The drawing under review shows one solid part. Ordinate dimensions are in mm from its lowest x, y, z. A direction names the side the tool comes from. Give positions to 0.01 mm unless a question says otherwise; leave off trailing zeros. Loops run counter-clockwise (first coordinate to the right, second up) from the corner with the lowest first, then second, coordinate; pieces in that order, holes last. Notation, with made-up numbers: M 37.5,19.5 L 92.5,19.5 A23 cw 92.5,45.5 Z; hole C 0,28 d9. An arc over 180 degrees is marked long. Write item = value, one per line. Start each with the question number.
1. For the marked faces 4, 5 and 6, list the 3-axis set-ups (+Z, -Z, +X, -X, +Y, -Y) from which the entire face can be reached by the end or side of a thin tool; tool diameter is ignored.
2. Draft analysis for pull direction Z (two halves, no side actions). For the marked faces 1, 2 and 3, state which applies: pulls with the +Z half, pulls with the -Z half, needs draft (parallel to the pull), parting line crosses it, or undercut.
3. Wall thickness on line 1 along Z through (x, y) = (2.25, 2); line 2 along Y through (x, z) = (21.75, 29.5); line 3 along Z through (x, y) = (21.75, 29) (1 decimal): over which ranges is each line inside the solid? List them lowest first. Write a range as from..to.
4. We need section A-A on y = 9. Give the boundary of the cut face in (x, z) (1 decimal).
5. For pin 1 (6 mm diameter, centred on x = 15, y = 7, fed in from -Z); pin 2 (1.5 mm diameter, centred on x = 18, z = 14, fed in from -Y); pin 3 (3.5 mm diameter, centred on x = 4.76, z = 4.76, fed in from +Y); pin 4 (4 mm diameter, centred on x = 10, z = 9.5, fed in from -Y), all flat-tipped, find the tip position at first contact; note any pin that passes through.
6. We need section B-B on z = 4.5. Give the boundary of the cut face in (x, y) (1 decimal), then the cut area to 3 significant figures.
7. We need section C-C on x = 20.5. Give the boundary of the cut face in (y, z) (1 decimal).
8. We need section D-D on z = 25. Give the boundary of the cut face in (x, y) (1 decimal).
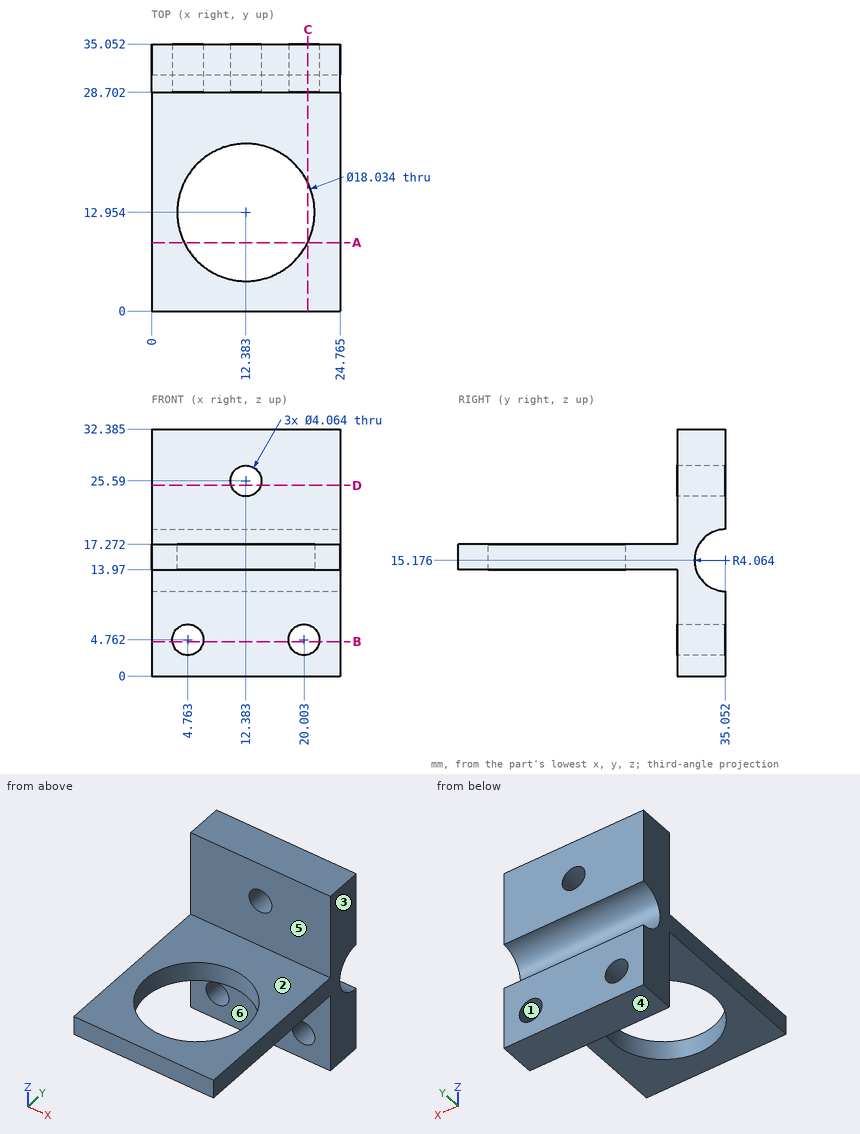
Final values:
q1.face_4 = -Z, +X, -X, +Y, -Y
q1.face_5 = +Z, +X, -X, -Y
q1.face_6 = -Z, +X, -X, -Y
q2.face_1 = undercut
q2.face_2 = pulls with the +Z half
q2.face_3 = needs draft
q3.line_1 = 13.97..17.27
q3.line_2 = 28.7..35.05
q3.line_3 = 0..3.7, 5.8..32.4
q4.outline = M 0,14 L 4.3,14 L 4.3,17.3 L 0,17.3 Z; M 20.5,14 L 24.8,14 L 24.8,17.3 L 20.5,17.3 Z
q5.pin_1 = 13.97
q5.pin_2 = 0
q5.pin_3 = through
q5.pin_4 = 28.7
q6.outline = M 0,28.7 L 2.7,28.7 L 2.7,35.1 L 0,35.1 Z; M 6.8,28.7 L 18,28.7 L 18,35.1 L 6.8,35.1 Z; M 22,28.7 L 24.8,28.7 L 24.8,35.1 L 22,35.1 Z
q6.area = 106 mm²
q7.outline = M 0,14 L 9,14 L 9,17.3 L 0,17.3 Z; M 16.9,14 L 28.7,14 L 28.7,6.7 L 35.1,6.7 L 35.1,11.1 A4.1 cw 35.1,19.2 L 35.1,32.4 L 28.7,32.4 L 28.7,17.3 L 16.9,17.3 Z; M 28.7,0 L 35.1,0 L 35.1,2.8 L 28.7,2.8 Z
q8.outline = M 0,28.7 L 10.4,28.7 L 10.4,35.1 L 0,35.1 Z; M 14.3,28.7 L 24.8,28.7 L 24.8,35.1 L 14.3,35.1 Z
